Here's how the part is built. I have some questions about the finished solid (model axes, mm). A direction names the side the tool comes from. Coordinates: 2 decimals unless noted, no trailing zeros. Loops run counter-clockwise (first coordinate to the right, second up) from the corner with the lowest first, then second, coordinate; pieces in that order, holes last. Notation, with made-up numbers: (46.5, 35) -> (82.5, 35) arc R17 cw to (82.5, 42) -> close; hole circle Ø8 at (66.25, 4.25). An arc over 180 degrees is marked (long way). Answer as a JSON object with one key per item and string values. Group by question number.
1) I want a section at C-C (x = 9.5). Write out the boundary of the cut face in (y, z).
2) I want a section at A-A (y = -2). Write out the boundary of the cut face in (x, z), then the cut area to 3 significant figures.
3) I need wall thicknesses on probe 1 along Y at (x, z) = (-22, -11.5); probe 2 along Z at (x, y) = (10, -1.05); probe 3 along X at (y, z) = (-2.05, 5.5). Which ranges of each line are inside material? Lowest first, please. Write a range as [from, to].
4) Which directions (+Z, -Z, +X, -X, +Y, -Y) give clear straight access to the entire face, cutting with the end or side of a thin tool? Please do faces 5 (the flat face through (-10.4, -1.27, 3.8)), 6 (the flat face through (0, -2.54, -14)).
5) I want a section at B-B (z = 5). Write out the boundary of the cut face in (x, y).
6) I'm going to push a flat-ended pin straight in: pin 1 (0.6 mm diameter, centred on x = -2, y = -2, fed in from +Z). Where does the tip first touch, or does it pass through?
7) If we mould it in two halves opening along Z, with no side actions, what happens to faces 1 (the flat face through (-11.438, -1.896, 6.979)), 2 (the cylindrical face through (10.331, -0.644, 3.253)), 3 (the flat face through (0, -1, -14.665)), 4 (the cylindrical face through (24.31, -1.29, -14.01))? For each: +Z half, -Z half, draft (parallel to the pull), parting line (faces both ways), or undercut.
8) I want a section at D-D (z = 12). Write out the boundary of the cut face in (x, y), then the cut area to 3 significant figures.
```python
from build123d import *

# Parameters (mm, degrees)
F1_DEPTH = 2.54
F2_R     = 1.27
F3_T     = 1.27
F4_R     = 10.8314490516
F5_DEPTH = 1.271


# Not quite as in the source:
# - a shell that OpenCascade refuses in one call is made with other operations: the cavity is built on its own and cut out


with BuildPart() as f1:
    # F0 (on Front) → F1 (new body)
    with BuildSketch(Plane.XZ):
        Polygon((25.4, -14.6646968374), (0, 29.3293936748), (-25.4, -14.6646968374), align=None)
    extrude(amount=F1_DEPTH)

    # F2
    f2_edges = [f1.edges().sort_by_distance(p)[0] for p in [
        (-25.4, -1.27, -14.664697),
        (25.4, -1.27, -14.664697),
        (0, -1.27, 29.329394),
    ]]
    fillet(f2_edges, radius=F2_R)

    # F3: shell of thickness 1.27, made by hand


with BuildPart() as f3_core1:
    # F3_t2: copy of F1
    add(f1.part)

    # the walls: a layer under each face that stays
    f3_faces = [f3_core1.faces().sort_by_distance(p)[0] for p in [
        (12.7, -1.27, 7.3323484187),
        (0, 0, 6.6973484187),
        (0, -1.27, -14.6646968374),
        (-12.7, -1.27, 7.3323484187),
    ]]
    thicken(f3_faces, amount=-F3_T, mode=Mode.SUBTRACT)


with BuildPart() as f1_1:
    add(f1.part)

    # what is left inside the walls is the cavity
    f3_cavity = [f3_core1.part.solids().sort_by_distance(p)[0] for p in [
        (0, -1.2827, 0),
    ]]
    add(f3_cavity, mode=Mode.SUBTRACT)

    # F4 (on face) → F5 (cut, through all)
    with BuildSketch(Plane.XZ.offset(1.27)):
        Circle(F4_R)
    extrude(amount=-F5_DEPTH, mode=Mode.SUBTRACT)


solid = f1_1.part
```
Determined:
{
 "1": {"outline": "(-2.54, -14.66) -> (0, -14.66) -> (0, -5.2) -> (-1.27, -5.2) -> (-1.27, -13.39) -> (-2.54, -13.39) -> close; (-2.54, 10.33) -> (-1.27, 10.33) -> (-1.27, 5.2) -> (0, 5.2) -> (0, 12.87) -> (-2.54, 12.87) -> close"},
 "2": {"outline": "(-24.3, -12.76) arc R1.27 ccw to (-23.2, -14.66) -> (23.2, -14.66) arc R1.27 ccw to (24.3, -12.76) -> (1.1, 27.42) arc R1.27 ccw to (-1.1, 27.42) -> close; hole (-23.2, -13.39) -> (23.2, -13.39) -> (0, 26.79) -> close", "area": "182 mm^2"},
 "3": {"probe 1": "[-1.27, 0]", "probe 2": "[-14.66, -4.16], [4.16, 12.01]", "probe 3": "[-13.76, -12.29], [12.29, 13.76]"},
 "4": {"face 5": "-Y", "face 6": "+Z, -Z, +X, -X, -Y"},
 "5": {"outline": "(-14.05, -2.54) -> (-12.58, -2.54) -> (-12.58, -1.27) -> (-9.61, -1.27) -> (-9.61, 0) -> (-14.05, 0) -> close; (9.61, -1.27) -> (12.58, -1.27) -> (12.58, -2.54) -> (14.05, -2.54) -> (14.05, 0) -> (9.61, 0) -> close"},
 "6": {"pin 1": "z = 26.38"},
 "7": {"face 1": "undercut", "face 2": "undercut", "face 3": "-Z half", "face 4": "parting line"},
 "8": {"outline": "(-10.01, -2.54) -> (-8.54, -2.54) -> (-8.54, -1.27) -> (8.54, -1.27) -> (8.54, -2.54) -> (10.01, -2.54) -> (10.01, 0) -> (-10.01, 0) -> close", "area": "29.1 mm^2"}
}
